Autodesk Inventor part; units mm, degrees
ref_plane "YZ Plane" through (0, 0, 0) normal (1, 0, 0) x (0, 1, 0)
ref_plane "XZ Plane" through (0, 0, 0) normal (0, 1, 0) x (-1, 0, 0)
ref_plane "XY Plane" through (0, 0, 0) normal (0, 0, 1) x (1, 0, 0)
sketch "Эскиз1" plane through (0, 0, 0) normal (0, 0, 1) x (1, 0, 0)
  line L0 (0, 0) -> (0, 49.2)
  line L1 (0, 49.2) -> (4.5, 49.2)
  line L2 (4.5, 49.2) -> (4.5, 46)
  line L3 (4.5, 46) -> (2, 46)
  line L4 (2, 46) -> (2, 6)
  line L5 (2, 6) -> (5, 6)
  line L6 (5, 6) -> (5, 0)
  line L7 (5, 0) -> (0, 0)
  dimension "d1" = 3
  dimension "d2" = 2.5
  dimension "d3" = 2
  dimension "d4" = 6
  dimension "d6" = 3.2
  dimension "d17" = 40
extrude "Выдавливание1" add sketch "Эскиз1" along normal blind 35
sketch "Эскиз2" plane through (5, 0, 0) normal (1, 0, 0) x (0, 0, -1)
  circle A0 centre (-24.5, 3) radius 1.4
  circle A1 centre (-10.5, 3) radius 1.4
  line L0 (0, 0) -> (-35, 0)
  line L1 (0, 0) -> (-35, 0)
  line L2 (0, 6) -> (-35, 6)
  point P0 (-17.5, 0)
  dimension "d9" = 2.8
  dimension "d10" = 2.8
  dimension "d11" = 14
  dimension "d12" = 7
  dimension "d13" = 3
  dimension "d14" = 6
extrude "Выдавливание2" cut sketch "Эскиз2" against normal blind 4.6
chamfer "Фаска1" distance 2.5 angle 45 1 edges at (4.5, 49.2, 17.5) measured on face at (4.5, 47.0667, 11.6667)
chamfer "Фаска2" distance 1 angle 60 4 edges at (0, 0, 17.5) (0, 49.2, 17.5) (0, 24.6, 0) (0, 24.6, 35) measured on face at (0, 32.8, 11.6667)
sketch "Эскиз3" plane through (2, 6, 0) normal (1, 0, 0) x (0, 0, -1)
  line L0 (-25, 5) -> (-10, 5)
  line L1 (-10, 5) -> (-10, 35)
  line L2 (-10, 35) -> (-25, 35)
  line L3 (-25, 35) -> (-25, 5)
  line L4 (-35, 0) -> (-35, 40)
  line L5 (0, 0) -> (0, 40)
  line L6 (0, 40) -> (-35, 40)
  point P0 (0, -6)
  dimension "d24" = 15
  dimension "d25" = 30
  dimension "d26" = 40
  dimension "d27" = 35
  dimension "d28" = 10
  dimension "d29" = 5
extrude "Выдавливание3" cut sketch "Эскиз3" against normal through all
chamfer "Фаска3" distance 0.5 angle 45 2 edges at (5, 3, 25.9) (5, 3, 11.9)
chamfer "Фаска4" distance 1 angle 60 4 edges at (0, 26, 10) (0, 11, 17.5) (0, 41, 17.5) (0, 26, 25) measured on face at (0, 20.0667, 31)
equation "\"d13\" = 0.5 * d14"
equation "\"d28\" = -0.5 * d24 + 0.5 * d27"
equation "\"d29\" = -0.5 * d25 + 0.5 * d26"
properties part number "Скоба"
Geometry check sheet. Reference: the model listing, model coordinates, mm. A direction names the side the tool comes from. Coordinates: 2 decimals unless noted, no trailing zeros. Order: outer loops, then holes, each group sorted by start corner. A loop starts at its lowest first (then second) coordinate and runs counter-clockwise, first axis right, second up. Notation, with made-up numbers: (-10.75, 13) - (44.25, 13) arc R8 cw to (44.25, 18) - close; hole circle Ø1 at (-33.75, 24). An arc over 180 degrees is marked (long way). Answer as a JSON object with one key per item and string values. Group by question number.
Item 1: Sectioned sample at B-B, the plane z = 10.5. Record the cut outline in (x, y), and give its area (3 significant figures).
Item 2: Depth check by flat-ended pin: pin 1 Ø10.5 at (y, z) = (30, 9.5) entering from +X; pin 2 Ø6 at (y, z) = (44.5, 3.5) entering from +X; pin 3 Ø2.5 at (y, z) = (3, 10.5) entering from +X. Enter the tip coordinate at first touch or a pass-through.
Item 3: Sectioned sample at C-C, the plane y = 19. Record the cut outline in (x, z).
Item 4: Draft check along Z on faces 1 (the face through (2.48, 2.15, 11.61)), 2 (the face through (2.48, 2.46, 23.21)), 3 (the face through (5, 3, 17)). Enter one of: +Z half, -Z half, draft (parallel to the pull), parting line (faces both ways), or undercut.
Item 5: Scan lines: probe 1 along Y at (x, z) = (3.05, 24.5); probe 2 along X at (y, z) = (43.5, 28.5); probe 3 along Z at (x, y) = (1.8, 25.5). Record each from-to range of solid material in increasing order.
Item 6: Tool access check on faces 4 (the face through (0.88, 26.22, 25.49)), 5 (the face through (3, 0, 17)), 6 (the face through (0.4, 3, 11)), 7 (the face through (2, 26, 9)), 8 (the face through (0.88, 0.49, 17.74)). Record the directions out of +Z, -Z, +X, -X, +Y, -Y that give a thin tool (end or side, any length) a straight path to the whole face; none if there is none.
Item 7: Sectioned sample at A-A, the plane x = 2.5. Record the cut outline in (y, z).
Item 8: Sectioned sample at D-D, the plane y = 3. Record the cut outline in (x, z).
Resolved:
{
 "1": {"outline": "(0, 1) - (1.73, 0) - (5, 0) - (5, 1.1) - (4.5, 1.6) - (0.4, 1.6) - (0.4, 4.4) - (4.5, 4.4) - (5, 4.9) - (5, 6) - (2, 6) - (2, 11) - (1.73, 11) - (0, 10) - close; (0, 42) - (1.73, 41) - (2, 41) - (2, 46) - (4.5, 46) - (4.5, 46.7) - (2, 49.2) - (1.73, 49.2) - (0, 48.2) - close", "area": "44.7 mm^2"},
 "2": {"pin 1": "x = 2", "pin 2": "x = 4.5", "pin 3": "x = 0.4"},
 "3": {"outline": "(0, 1) - (1.73, 0) - (2, 0) - (2, 10) - (1.73, 10) - (0, 9) - close; (0, 26) - (1.73, 25) - (2, 25) - (2, 35) - (1.73, 35) - (0, 34) - close"},
 "4": {"face 1": "undercut", "face 2": "undercut", "face 3": "draft"},
 "5": {"probe 1": "0 to 1.6, 4.4 to 6, 46 to 48.15", "probe 2": "0 to 2", "probe 3": "0 to 10, 25 to 35"},
 "6": {"face 4": "-X", "face 5": "+Z, -Z, +X, -X, -Y", "face 6": "+X", "face 7": "+Z, -Z, +X", "face 8": "+Z, -Z, -X, -Y"},
 "7": {"outline": "(0, 0) - (6, 0) - (6, 35) - (0, 35) - close; (46, 0) - (48.7, 0) - (48.7, 35) - (46, 35) - close; hole circle Ø2.8 at (3, 10.5); hole circle Ø2.8 at (3, 24.5)"},
 "8": {"outline": "(0, 1) - (1.73, 0) - (5, 0) - (5, 8.6) - (4.5, 9.1) - (0.4, 9.1) - (0.4, 11.9) - (4.5, 11.9) - (5, 12.4) - (5, 22.6) - (4.5, 23.1) - (0.4, 23.1) - (0.4, 25.9) - (4.5, 25.9) - (5, 26.4) - (5, 35) - (1.73, 35) - (0, 34) - close"}
}
